Verification items for the finished model (mm, model axes). A direction names the side the tool comes from. Round coordinates to 2 decimals unless told otherwise and drop trailing zeros. Loops run counter-clockwise (first coordinate to the right, second up) from the corner with the lowest first, then second, coordinate; pieces in that order, holes last.
from build123d import *

# Parameters (mm, degrees)
SKETCH1_W           = 60
SKETCH1_H           = 35
BOSS_EXTRUDE1_DEPTH = 18
SKETCH2_R           = 3.1
CUT_EXTRUDE1_DEPTH  = 18
SKETCH3_R           = 1.45
SKETCH3_W           = 36.5
SKETCH3_H           = 26
CUT_EXTRUDE2_DEPTH  = 11
SKETCH4_R           = 2.975
BOSS_EXTRUDE2_DEPTH = 11
SKETCH6_R           = 1
CUT_EXTRUDE3_DEPTH  = 5.8
SKETCH8_R           = 1
CUT_EXTRUDE4_DEPTH  = 5.8
FILLET2_R           = 0.5


with BuildPart() as part:
    # Sketch1 → Boss-Extrude1 (new body)
    with BuildSketch(Plane.XY):
        with Locations((30, 17.5)):
            Rectangle(SKETCH1_W, SKETCH1_H)
    extrude(amount=BOSS_EXTRUDE1_DEPTH)

    # Sketch2 → Cut-Extrude1 (cut)
    with BuildSketch(Plane.XY.offset(18)):
        with Locations((11.25, 26)):
            Circle(SKETCH2_R)
        with Locations((11.25, 9)):
            Circle(SKETCH2_R)
    extrude(amount=-CUT_EXTRUDE1_DEPTH, mode=Mode.SUBTRACT)

    # Sketch3 → Cut-Extrude2 (cut)
    with BuildSketch(Plane.XY.offset(18)):
        with Locations((3, 32)):
            Circle(SKETCH3_R)
        with Locations((57, 32)):
            Circle(SKETCH3_R)
        with Locations((57, 3)):
            Circle(SKETCH3_R)
        with Locations((3, 3)):
            Circle(SKETCH3_R)
        with Locations((36.25, 17.5)):
            Rectangle(SKETCH3_W, SKETCH3_H)
    extrude(amount=-CUT_EXTRUDE2_DEPTH, mode=Mode.SUBTRACT)

    # Sketch4 → Boss-Extrude2 (add)
    with BuildSketch(Plane.XY.offset(7)):
        with Locations(Location((36.25, 15, 0), (0, 0, 180))):
            Circle(SKETCH4_R)
        with Locations(Location((47.5, 20, 0), (0, 0, 180))):
            Circle(SKETCH4_R)
    extrude(amount=BOSS_EXTRUDE2_DEPTH)

    # Sketch6 → Cut-Extrude3 (cut)
    with BuildSketch(Plane(origin=(60, 0, 0), x_dir=(0, 0, -1), z_dir=(1, 0, 0))):
        with Locations((-9, 20.475)):
            Circle(SKETCH6_R)
    extrude(amount=-CUT_EXTRUDE3_DEPTH, mode=Mode.SUBTRACT)

    # Sketch8 → Cut-Extrude4 (cut)
    with BuildSketch(Plane.XZ):
        with Locations(Location((22.025, 9, 0), (0, 0, 270))):
            Circle(SKETCH8_R)
    extrude(amount=-CUT_EXTRUDE4_DEPTH, mode=Mode.SUBTRACT)

    # Fillet2
    fillet2_edges = [part.edges().sort_by_distance(p)[0] for p in [
        (54.5, 20.475, 10),
        (60, 20.475, 10),
        (22.025, 4.5, 10),
        (22.025, 0, 10),
    ]]
    fillet(fillet2_edges, radius=FILLET2_R)


solid = part.part
1. Gauge pin test, flat ends, axial feed: P1, Ø1.7, axis at x = 57, y = 32, coming from the +Z side; P2, Ø2, axis at y = 16.5, z = 11.5, coming from the -X side; P3, Ø3.5, axis at x = 11.25, y = 26, coming from the +Z side; P4, Ø1.8, axis at x = 22.025, z = 9, coming from the -Y side. Record the tip position at first contact, or that the pin passes through.
2. Section check C-C (x = 11.25). Enter the section's corners in (y, z), then the cut area to 3 significant figures.
3. Release check for a two-part mould opening along Y. For faces 4 (the face through (57, 3, 7)), 5 (the face through (30, 35, 9)), 6 (the face through (23.016, 2.226, 9.13)) record: released by +Y, released by -Y, zero draft, split by the parting line, or undercut.
4. Scan lines: L1, parallel to Y at x = 3, z = 12.5; L2, parallel to Y at x = 11.25, z = 11.5; L3, parallel to X at y = 30, z = 13. Record each from-to range of solid material in increasing order.
5. Tool access check on faces 1 (the face through (48.145, 22.904, 12.423)), 2 (the face through (0, 17, 9)), 3 (the face through (57.282, 19.867, 9.794)). Record the directions out of +Z, -Z, +X, -X, +Y, -Y that give a thin tool (end or side, any length) a straight path to the whole face; none if there is none.
6. Section check A-A (y = 26). Enter the section's corners in (x, z), then the cut area to 3 significant figures.
7. Section check B-B (z = 9). Give the number of separate pieces and of enclosed holes in the cut face, then the cut area to 3 significant figures.
Taken from the geometry:
1. P1: stops at z = 7
1. P2: stops at x = 0
1. P3: passes through
1. P4: stops at y = 30.5
2. outline: (0, 0) - (5.9, 0) - (5.9, 18) - (0, 18) - close; (12.1, 0) - (22.9, 0) - (22.9, 18) - (12.1, 18) - close; (29.1, 0) - (35, 0) - (35, 18) - (29.1, 18) - close
2. area: 407 mm2
3. face 4: undercut
3. face 5: released by +Y
3. face 6: zero draft
4. L1: y = 0 to 1.55, 4.45 to 30.55, 33.45 to 35
4. L2: y = 0 to 5.9, 12.1 to 22.9, 29.1 to 35
4. L3: x = 0 to 18, 54.5 to 60
5. face 1: +Z
5. face 2: +Z, -Z, -X, +Y, -Y
5. face 3: +X
6. outline: (0, 0) - (8.15, 0) - (8.15, 18) - (0, 18) - close; (14.35, 0) - (60, 0) - (60, 18) - (54.5, 18) - (54.5, 7) - (18, 7) - (18, 18) - (14.35, 18) - close
6. area: 567 mm2
7. separate pieces: 4
7. enclosed holes: 6
7. area: 1,100 mm2
